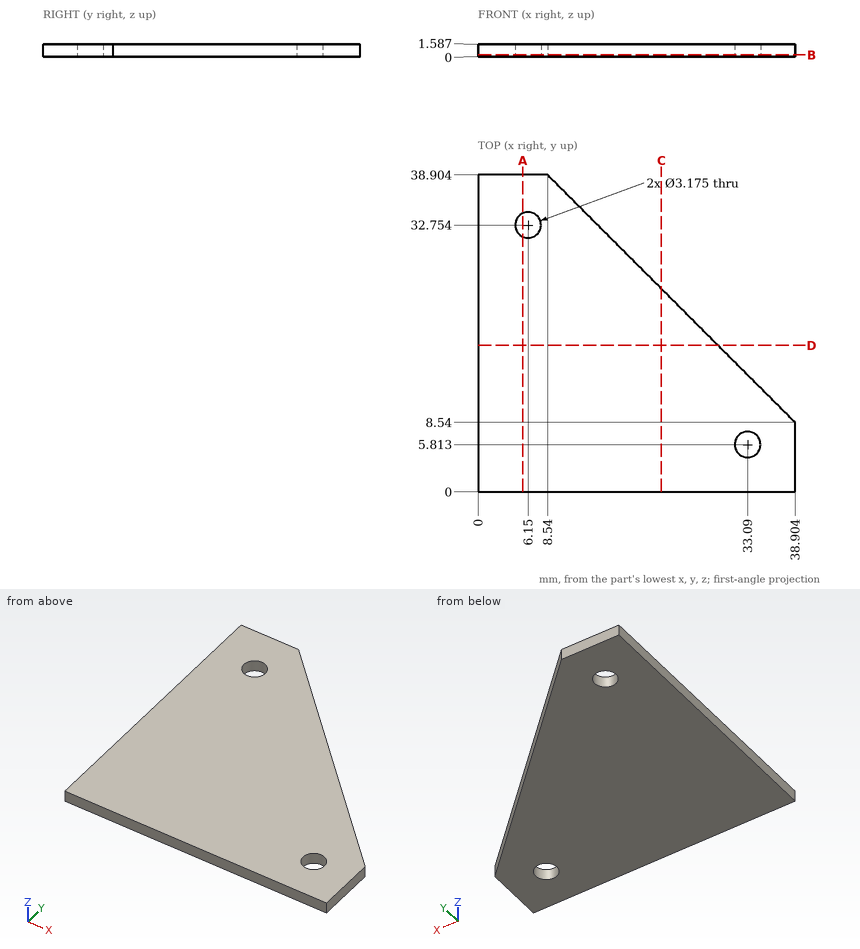
Source: three-view drawing plus pictorial views. Frame: mm from the lowest corner of the part. Round coordinates to 2 decimals unless told otherwise and drop trailing zeros. Loops run counter-clockwise (first coordinate to the right, second up) from the corner with the lowest first, then second, coordinate; pieces in that order, holes last.
1. Section query A-A on x = 5.5. Output: boundary loops of the cut face in (y, z) (1 decimal).
2. Contact query for a flat-ended pin moving along its axis: pin 1 (5 mm diameter, centred on x = 6.15, y = 32.75, fed in from -Z). Output: stop coordinate, or through.
3. Ray query, L1, parallel to Y at x = 6, z = 0.15 (1 decimal); L2, parallel to X at y = 6, z = 0.2 (1 decimal); L3, parallel to X at y = 7, z = 0.5 (1 decimal). Return the intervals inside material, ascending.
4. Section query B-B on z = 0.25. Give the number of separate pieces and of enclosed holes in the cut face, and give its area (3 significant figures).
5. Section query D-D on y = 18. Output: boundary loops of the cut face in (x, z).
6. Section query C-C on x = 22.5. Output: boundary loops of the cut face in (y, z).
Answers below:
1. outline: (0, 0) - (31.3, 0) - (31.3, 1.6) - (0, 1.6) - close; (34.2, 0) - (38.9, 0) - (38.9, 1.6) - (34.2, 1.6) - close
2. pin 1: stops at z = 0
3. L1: y = 0 to 31.2, 34.3 to 38.9
3. L2: x = 0 to 31.5, 34.7 to 38.9
3. L3: x = 0 to 32, 34.1 to 38.9
4. separate pieces: 1
4. enclosed holes: 2
4. area: 1,040 mm2
5. outline: (0, 0) - (29.44, 0) - (29.44, 1.59) - (0, 1.59) - close
6. outline: (0, 0) - (24.94, 0) - (24.94, 1.59) - (0, 1.59) - close
